```python
from build123d import *

# Parameters (mm, degrees)
SKETCH18_W                     = 148
SKETCH18_H                     = 205.5334
BASE_FLANGE1_DEPTH             = 3
EDGE_FLANGE1_STRIP_W           = 13.4732
EDGE_FLANGE1_STRIP_H           = 3
EDGE_FLANGE1_STRIP_CUT_DEPTH   = 205.5334
EDGE_FLANGE1_STRIP_2_W         = 13.4732
EDGE_FLANGE1_STRIP_2_H         = 3
EDGE_FLANGE1_STRIP_CUT_2_DEPTH = 205.5334
EDGE_FLANGE1_DEPTH             = 205.5334
EDGE_FLANGE1_BEND_DEPTH        = 205.5334
SKETCH28_W                     = 150
SKETCH28_H                     = 8
CUT_EXTRUDE2_DEPTH             = 25
SKETCH30_R                     = 3
CUT_EXTRUDE3_DEPTH             = 225.935458149
SKETCH31_W                     = 157.455262849
SKETCH31_H                     = 40
CUT_EXTRUDE4_DEPTH             = 10
CHAMFER1_SIZE                  = 5


# Sheet-metal steps are written as plain solids
with BuildPart() as part:
    # Sketch18 → Base-Flange1 (new body)
    with BuildSketch(Plane(origin=(0, 0, 0), x_dir=(1, 0, 0), z_dir=(0, 1, 0))):
        with Locations((-74, -63.57018807)):
            Rectangle(SKETCH18_W, SKETCH18_H)
    extrude(amount=-BASE_FLANGE1_DEPTH)

    # Edge-Flange1 strip (across the edge) → Edge-Flange1 strip cut (cut)
    with BuildSketch(Plane(origin=(0, 0, 166.33688807), x_dir=(-1, 0, 0), z_dir=(0, 0, -1))):
        with Locations((-3, -1.5)):
            Rectangle(EDGE_FLANGE1_STRIP_W, EDGE_FLANGE1_STRIP_H)
    extrude(amount=EDGE_FLANGE1_STRIP_CUT_DEPTH, mode=Mode.SUBTRACT)

    # Edge-Flange1 strip 2 (across the edge) → Edge-Flange1 strip cut 2 (cut)
    with BuildSketch(Plane(origin=(-148, 0, -39.19651193), x_dir=(1, 0, 0), z_dir=(0, 0, 1))):
        with Locations((-3, -1.5)):
            Rectangle(EDGE_FLANGE1_STRIP_2_W, EDGE_FLANGE1_STRIP_2_H)
    extrude(amount=EDGE_FLANGE1_STRIP_CUT_2_DEPTH, mode=Mode.SUBTRACT)

    # Edge-Flange1 section (across the edge) → Edge-Flange1 (add)
    with BuildSketch(Plane(origin=(0, 0, 166.33688807), x_dir=(-1, 0, 0), z_dir=(0, 0, -1))):
        with BuildLine():
            Line((0, 0.7366), (0, 32))
            Line((0, 32), (3, 32))
            Line((3, 32), (3, 0.7366))
            ThreePointArc((3, 0.7366), (3.215745145, 0.215745145), (3.7366, 0))
            Line((3.7366, 0), (3.7366, -3))
            ThreePointArc((3.7366, -3), (1.094424801, -1.905575199), (0, 0.7366))
        make_face()
    extrude(amount=EDGE_FLANGE1_DEPTH)

    # Edge-Flange1 section 2 (across the edge) → Edge-Flange1 bend (add)
    with BuildSketch(Plane(origin=(-148, 0, -39.19651193), x_dir=(1, 0, 0), z_dir=(0, 0, 1))):
        with BuildLine():
            Line((0, 0.7366), (0, 32))
            Line((0, 32), (3, 32))
            Line((3, 32), (3, 0.7366))
            ThreePointArc((3, 0.7366), (3.215745145, 0.215745145), (3.7366, 0))
            Line((3.7366, 0), (3.7366, -3))
            ThreePointArc((3.7366, -3), (1.094424801, -1.905575199), (0, 0.7366))
        make_face()
    extrude(amount=EDGE_FLANGE1_BEND_DEPTH)

    # Sketch28 → Cut-Extrude2 (cut)
    with BuildSketch(Plane.XY.offset(166.33688807)):
        with Locations((-74, -2)):
            Rectangle(SKETCH28_W, SKETCH28_H)
    extrude(amount=-CUT_EXTRUDE2_DEPTH, mode=Mode.SUBTRACT)

    # Sketch30 → Cut-Extrude3 (cut, through all)
    with BuildSketch(Plane.ZY.offset(148)):
        with Locations(Location((152.33688807, 14.23, 0), (0, 0, 270))):
            Circle(SKETCH30_R)
        with Locations(Location((-19.66651193, 18.64, 0), (0, 0, 270))):
            Circle(SKETCH30_R)
    extrude(amount=-CUT_EXTRUDE3_DEPTH, mode=Mode.SUBTRACT)

    # Sketch31 → Cut-Extrude4 (cut)
    with BuildSketch(Plane(origin=(0, 0, -39.19651193), x_dir=(-1, 0, 0), z_dir=(0, 0, -1))):
        with Locations((75.148815223, 17)):
            Rectangle(SKETCH31_W, SKETCH31_H)
    extrude(amount=-CUT_EXTRUDE4_DEPTH, mode=Mode.SUBTRACT)

    # Chamfer1
    chamfer1_edges = [part.edges().sort_by_distance(p)[0] for p in [
        (-1.5, 2, 166.33688807),
        (-146.5, 32, -29.19651193),
        (-1.5, 32, -29.19651193),
        (-1.5, 32, 166.33688807),
        (-146.5, 32, 166.33688807),
        (-146.5, 2, 166.33688807),
    ]]
    chamfer(chamfer1_edges, length=CHAMFER1_SIZE)


solid = part.part
```
Design review of the part built by this model. Coordinates are the model's own, in mm. A direction names the side the tool comes from. Round coordinates to 2 decimals unless told otherwise and drop trailing zeros. Write each loop counter-clockwise with the first axis right and the second up, starting at its lowest first coordinate (ties: lowest second). Pieces come first, ordered by that corner, then holes.
Item 1: For faces 1 (the flat face through (-148, 16, 67)), 2 (the flat face through (-3, 17, 70)), list the 3-axis set-ups (+Z, -Z, +X, -X, +Y, -Y) from which the entire face can be reached by the end or side of a thin tool; tool diameter is ignored.
Item 2: We need section C-C on x = -129.5. Write out the cut boundary in (y, z).
Item 3: For probe 1 along X at (y, z) = (9, 133.5); probe 2 along Y at (x, z) = (-137, 85); probe 3 along Z at (x, y) = (-139, -0.5), list the stretches that pass through material, from the lowest coordinate up.
Item 4: We need section A-A on z = 113.5. Write out the cut boundary in (x, y).
Item 5: We need section B-B on y = 5. Write out the cut boundary in (x, z), and give its area (3 significant figures).
Item 6: The part is to be moulded in two halves that separate along X. For faces 3 (the cylindrical face through (-146.88, -1.93, 54.88)), 4 (the flat face through (-145, 17, 67)), 5 (the flat face through (-1.479, 29.465, 163.872)), say which applies: +X half, -X half, draft (parallel to the pull), parting line (faces both ways), or undercut.
Item 7: Clearance check with flat-ended pins moving along their axes: pin 1 Ø2.5 at (x, z) = (-146.5, 156) entering from -Y; pin 2 Ø5 at (y, z) = (14.23, 152.34) entering from -X; pin 3 Ø4 at (x, y) = (-74, -1.5) entering from +Z; pin 4 Ø12 at (x, z) = (-52.5, 109.5) entering from +Y. State where each tip first meets the part, or that it passes through.
Returned:
1. face 1: +Z, -Z, -X, +Y, -Y
1. face 2: +Z, -Z, +Y
2. outline: (-3, -29.2) - (0, -29.2) - (0, 141.34) - (-3, 141.34) - close
3. probe 1: x = -148 to -145, -3 to 0
3. probe 2: y = -3 to 0
3. probe 3: z = -29.2 to 141.34
4. outline: (-148, 0.74) arc R3.74 ccw to (-144.26, -3) - (-3.74, -3) arc R3.74 ccw to (0, 0.74) - (0, 32) - (-3, 32) - (-3, 0.74) arc R0.74 cw to (-3.74, 0) - (-144.26, 0) arc R0.74 cw to (-145, 0.74) - (-145, 32) - (-148, 32) - close
5. outline: (-148, -29.2) - (-145, -29.2) - (-145, 164.34) - (-148, 164.34) - close; (-3, -29.2) - (0, -29.2) - (0, 164.34) - (-3, 164.34) - close
5. area: 1,160 mm2
6. face 3: -X half
6. face 4: undercut
6. face 5: draft
7. pin 1: stops at y = 2
7. pin 2: passes through
7. pin 3: stops at z = 141.34
7. pin 4: stops at y = 0
